```python
from build123d import *

# Parameters (mm, degrees)
BOSS_EXTRUDE2_DEPTH = 10
SKETCH2_R           = 0.5
CUT_EXTRUDE1_DEPTH  = 15.57614975
LPATTERN1_COUNT     = 2
LPATTERN1_PITCH     = 5


with BuildPart() as part:
    # Sketch1 → Boss-Extrude2 (new body)
    with BuildSketch(Plane(origin=(0, 0, 0), x_dir=(1, 0, 0), z_dir=(0, 1, 0))):
        Polygon((-12.31884058, 7.632850242), (-12.31884058, -2.367149758), (-11.31884058, -2.367149758), (-11.31884058, 1.632850242), (-5.956521739, 1.632850242), (-5.956521739, -2.367149758), (-4.956521739, -2.367149758), (-4.956521739, 7.632850242), (-5.956521739, 7.632850242), (-5.956521739, 3.632850242), (-11.31884058, 3.632850242), (-11.31884058, 7.632850242), align=None)
    extrude(amount=BOSS_EXTRUDE2_DEPTH)

    # Sketch2 → Cut-Extrude1 (cut, through all)
    with BuildSketch(Plane(origin=(-4.956521739, 0, 0), x_dir=(0, 0, -1), z_dir=(1, 0, 0))):
        with Locations((0, 5)):
            Circle(SKETCH2_R)
    cut_extrude1 = extrude(amount=-CUT_EXTRUDE1_DEPTH, mode=Mode.SUBTRACT)

    # LPattern1: Cut-Extrude1 ×2
    with Locations(*[(0, 0, -i * LPATTERN1_PITCH) for i in range(1, LPATTERN1_COUNT)]):
        add(cut_extrude1, mode=Mode.SUBTRACT)


solid = part.part
```
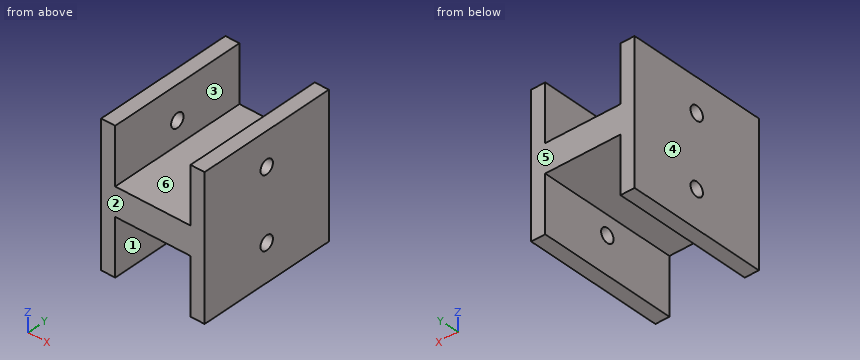
The listing builds one solid part. Answer for the finished solid, in the listing's coordinates (mm). Face numbers are marked on the shaded views. A direction names the side the tool comes from. Coordinates: 2 decimals unless noted, no trailing zeros. Write each loop counter-clockwise with the first axis right and the second up, starting at its lowest first coordinate (ties: lowest second). Pieces come first, ordered by that corner, then holes. Notation, with made-up numbers: M -20.75,22 L -14.75,22 A24 cw -14.75,57 Z; hole C 41,87.25 d11. An arc over 180 degrees is marked long. Use a Markdown table: item, result. Add a question column.
1. Given P1, Ø2, axis at x = -9.5, z = 0.5, coming from the +Y side; P2, Ø3, axis at x = -8, y = 5.5, coming from the -Z side; P3, Ø4, axis at x = -9, y = 2, coming from the +Z side, each flat-ended and moving along its own axis, determine where each tip first touches the part or whether it passes through.
2. Straight lines are drawn through the part: line 1 along Y through (x, z) = (-12.1, -5); line 2 along X through (y, z) = (4, 1.5); line 3 along Z through (x, y) = (-9.25, 8). For each, find the intervals that lie inside material, in ascending order. Write a range as [from, to].
3. Section A-A (y = 5) is taken. Give the vertices of the cut face in (x, z), plus the area to 3 significant figures.
4. Which of the six approach directions +Z, -Z, +X, -X, +Y, -Y give full straight-line access (tool end or side, diameter ignored) to the marked faces 1, 2 and 3?
5. Section D-D (y = 1.75) is taken. Give the vertices of the cut face in (x, z), plus the area to 3 significant figures.
6. For a pull along X with two mould halves and no side action, classify the marked faces 4, 5 and 6 as +X half, -X half, draft (parallel to the pull), parting line (faces both ways), or undercut.
7. Section C-C (x = -5.25) is taken. Give the vertices of the cut face in (y, z).
8. Section B-B (z = 0.75) is taken. Give the vertices of the cut face in (x, y).
Data:
| question | item | result |
|---|---|---|
| 1 | P1 | passes through |
| 1 | P2 | stops at z = -3.63 |
| 1 | P3 | stops at z = -1.63 |
| 2 | line 1 | y = [0, 4.5], [5.5, 10] |
| 2 | line 2 | x = [-12.32, -11.32], [-5.96, -4.96] |
| 2 | line 3 | z = [-3.63, -1.63] |
| 3 | outline | M -12.32,-7.63 L -11.32,-7.63 L -11.32,-5.5 L -12.32,-5.5 Z; M -12.32,-4.5 L -11.32,-4.5 L -11.32,-3.63 L -5.96,-3.63 L -5.96,-4.5 L -4.96,-4.5 L -4.96,-0.5 L -5.96,-0.5 L -5.96,-1.63 L -11.32,-1.63 L -11.32,-0.5 L -12.32,-0.5 Z; M -12.32,0.5 L -11.32,0.5 L -11.32,2.37 L -12.32,2.37 Z; M -5.96,-7.63 L -4.96,-7.63 L -4.96,-5.5 L -5.96,-5.5 Z; M -5.96,0.5 L -4.96,0.5 L -4.96,2.37 L -5.96,2.37 Z |
| 3 | area | 26.7 mm2 |
| 4 | face 1 | -Z, +Y, -Y |
| 4 | face 2 | +Z, -Z, +X, -X, -Y |
| 4 | face 3 | +Z, +Y, -Y |
| 5 | outline | M -12.32,-7.63 L -11.32,-7.63 L -11.32,-3.63 L -5.96,-3.63 L -5.96,-7.63 L -4.96,-7.63 L -4.96,2.37 L -5.96,2.37 L -5.96,-1.63 L -11.32,-1.63 L -11.32,2.37 L -12.32,2.37 Z |
| 5 | area | 30.7 mm2 |
| 6 | face 4 | -X half |
| 6 | face 5 | draft |
| 6 | face 6 | undercut |
| 7 | outline | M 0,-7.63 L 10,-7.63 L 10,2.37 L 0,2.37 Z; hole C 5,-5 d1; hole C 5,0 d1 |
| 8 | outline | M -12.32,0 L -11.32,0 L -11.32,10 L -12.32,10 Z; M -5.96,0 L -4.96,0 L -4.96,10 L -5.96,10 Z |
